Could you check a few things on this model? Use its own coordinates, in mm. Face numbers are marked on the shaded views. A direction names the side the tool comes from. Round coordinates to 2 decimals unless told otherwise and drop trailing zeros. Loops run counter-clockwise (first coordinate to the right, second up) from the corner with the lowest first, then second, coordinate; pieces in that order, holes last. Notation, with made-up numbers: (38.25, 1) -> (67.25, 1) arc R17 ccw to (67.25, 14) -> close; hole circle Ø2 at (20.5, 9.25). An arc over 180 degrees is marked (long way). Put each result on its own line as item: value. Start each with the question number.
1. I need wall thicknesses on line 1 (X direction, y = 5, z = -14); line 2 (Z direction, x = 5.5, y = -3.75). Which ranges of each line are inside material? Lowest first, please. Write a range as [from, to].
2. Which directions (+Z, -Z, +X, -X, +Y, -Y) give clear straight access to the entire face, cutting with the end or side of a thin tool? Please do the marked faces 4 and 5.
3. Imagine slicing it at B-B, the plane y = 5.25. Please give me the cut outline in (x, z), and give its area (3 significant figures).
4. Imagine slicing it at C-C, the plane x = 0.5. Please give me the cut outline in (y, z), and give its area (3 significant figures).
5. If we mould it in two halves opening along X, with no side actions, what happens to the marked faces 1, 2 and 3? For each: pulls with the +X half, pulls with the -X half, needs draft (parallel to the pull), parting line crosses it, or undercut.
6. I'm going to push a flat-ended pin straight in: P1, Ø4, axis at x = -1.5, y = -1.5, coming from the -Z side. Where does the tip first touch, or does it pass through?
7. Imagine slicing it at A-A, the plane z = -8.5. Please give me the cut outline in (x, y).
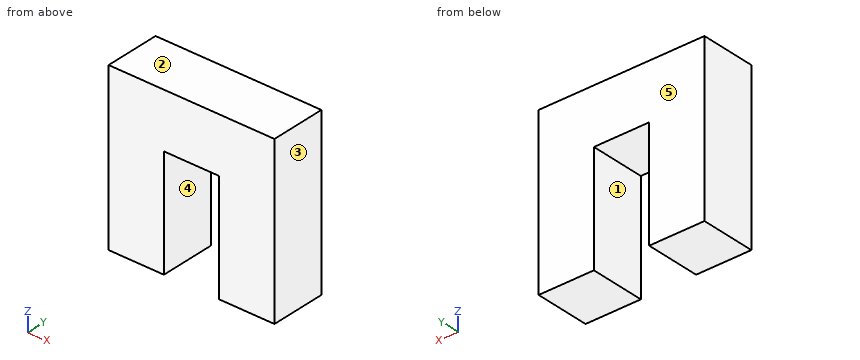
```python
from build123d import *

# Parameters (mm, degrees)
F0_W     = 12.7
F0_H     = 12.7
F1_DEPTH = 6.35


with BuildPart() as f1:
    # F0 (on Front) → F1 (new body, symmetric)
    with BuildSketch(Plane.XZ):
        with Locations((-12.7, 10.885714)):
            Rectangle(F0_W, F0_H)
        with Locations((0, 10.885714)):
            Rectangle(F0_W, F0_H)
        with Locations((-12.7, -1.814286)):
            Rectangle(F0_W, F0_H)
        with Locations((12.7, 10.885714)):
            Rectangle(F0_W, F0_H)
        with Locations((-12.7, -14.514286)):
            Rectangle(F0_W, F0_H)
        with Locations((12.7, -1.814286)):
            Rectangle(F0_W, F0_H)
        with Locations((12.7, -14.514286)):
            Rectangle(F0_W, F0_H)
    extrude(amount=F1_DEPTH, both=True)


solid = f1.part
```
Entries:
1. line 1: [-19.05, -6.35], [6.35, 19.05]
1. line 2: [4.54, 17.24]
2. face 4: -Z, +Y, -Y
2. face 5: +Z, -Z, +X, -X, +Y
3. outline: (-19.05, -20.86) -> (-6.35, -20.86) -> (-6.35, 4.54) -> (6.35, 4.54) -> (6.35, -20.86) -> (19.05, -20.86) -> (19.05, 17.24) -> (-19.05, 17.24) -> close
3. area: 1,130 mm^2
4. outline: (-6.35, 4.54) -> (6.35, 4.54) -> (6.35, 17.24) -> (-6.35, 17.24) -> close
4. area: 161 mm^2
5. face 1: undercut
5. face 2: needs draft
5. face 3: pulls with the +X half
6. P1: z = 4.54
7. outline: (-19.05, -6.35) -> (-6.35, -6.35) -> (-6.35, 6.35) -> (-19.05, 6.35) -> close; (6.35, -6.35) -> (19.05, -6.35) -> (19.05, 6.35) -> (6.35, 6.35) -> close
